Read the model definition and answer for the solid it produces. Units are mm, in the model's axes. A direction names the side the tool comes from. Coordinates: 2 decimals unless noted, no trailing zeros. Loops run counter-clockwise (first coordinate to the right, second up) from the corner with the lowest first, then second, coordinate; pieces in that order, holes last. Notation, with made-up numbers: (-12.75, 55) - (-8.75, 55) arc R29 cw to (-8.75, 88) - close; hole circle Ø11 at (27.25, -36). An arc over 180 degrees is marked (long way). One line per question, with ' | ' between items. Start each with the question number.
```python
from build123d import *

# Parameters (mm, degrees)
F0_R     = 2
F1_DEPTH = 20
F2_W     = 1
F2_H     = 5.5
F3_DEPTH = 10
F4_R     = 1.5
F5_DEPTH = 26.301
F6_SIZE  = 0.5
F7_R     = 1
F9_DEPTH = 3


with BuildPart() as f1:
    # F0 (on Top) → F1 (new body)
    with BuildSketch(Plane.XY):
        with BuildLine():
            Line((0, 3), (0, 0))
            Line((0, 0), (10, 0))
            ThreePointArc((10, 0), (23.15, 13.15), (10, 26.3))
            Line((10, 26.3), (0, 26.3))
            Line((0, 26.3), (0, 23.3))
            Line((0, 23.3), (10, 23.3))
            Line((10, 23.3), (10, 3))
            Line((10, 3), (0, 3))
        make_face()
        with Locations((17, 13.15)):
            Circle(F0_R, mode=Mode.SUBTRACT)
    extrude(amount=F1_DEPTH)

    # F2 (on face) → F3 (join, through all)
    with BuildSketch(Plane(origin=(10, 0, 0), x_dir=(0, -1, 0), z_dir=(-1, 0, 0))):
        with Locations((-22.8, 10)):
            Rectangle(F2_W, F2_H)
        with Locations((-3.5, 10)):
            Rectangle(F2_W, F2_H)
    extrude(amount=F3_DEPTH)

    # F4 (on face) → F5 (cut, through all)
    with BuildSketch(Plane.XZ):
        with Locations((5, 10)):
            Circle(F4_R)
    extrude(amount=-F5_DEPTH, mode=Mode.SUBTRACT)

    # F6
    f6_edges = [f1.edges().sort_by_distance(p)[0] for p in [
        (15, 13.15, 0),
    ]]
    chamfer(f6_edges, length=F6_SIZE)

    # F7
    f7_edges = [f1.edges().sort_by_distance(p)[0] for p in [
        (23.15, 13.15, 20),
        (23.15, 13.15, 0),
        (0, 0, 10),
        (0, 26.3, 10),
    ]]
    fillet(f7_edges, radius=F7_R)

    # F8 (on face) → F9 (cut)
    with BuildSketch(Plane.XY.offset(20)):
        Polygon((20.75, 10.984936), (20.75, 15.315064), (17, 17.480127), (13.25, 15.315064), (13.25, 10.984936), (17, 8.819873), align=None)
    extrude(amount=-F9_DEPTH, mode=Mode.SUBTRACT)


solid = f1.part
```
1) Which of the six approach directions +Z, -Z, +X, -X, +Y, -Y give full straight-line access (tool end or side, diameter ignored) to faces 4 (the flat face through (5.1, 3.5, 12.75)), 5 (the flat face through (5, 23.3, 4)), 6 (the flat face through (0, 24, 10)), 7 (the flat face through (13.25, 13, 19)), 8 (the flat face through (6.2, 4, 11.2))?
2) The mould has two halves that part along X. Classify faces 1 (the flat face through (0, 2, 10)), 2 (the flat face through (15.15, 16.41, 18.52)), 3 (the flat face through (5, 3, 16)): released by +X, released by -X, zero draft, split by the parting line, or undercut.
3) Given pin 1 Ø1 at (y, z) = (7.5, 14.5) entering from +X; pin 2 Ø5 at (x, z) = (5, 10) entering from -Y; pin 3 Ø2.5 at (x, z) = (5, 10) entering from -Y; pin 4 Ø4.5 at (x, y) = (17, 13.15) entering from -Z, each flat-ended and moving along its own axis, determine where each tip first touches the part or whether it passes through.
4) Find the intervals of material crossed by line 1 along Z through (x, y) = (5, 1.6); line 2 along X through (y, z) = (13.15, 13); line 3 along Y through (x, z) = (5.75, 2), in increasing order. Write a range as from..to.
5) The part is cut by section C-C on z = 2.25. Write down the section's boundary in (x, y), and give its area (3 significant figures).
6) The part is cut by section D-D on x = 5. Write down the section's boundary in (y, z).
7) The part is cut by section A-A on x = 2. Write down the section's boundary in (y, z).
8) The part is cut by section B-B on y = 13.15. Write down the section's boundary in (x, z), and give its area (3 significant figures).
Answer below:
1) face 4: +Z, -X | face 5: -Z, -X | face 6: +Z, -Z, -X, +Y, -Y | face 7: +Z | face 8: +Z, -Z, -X
2) face 1: released by -X | face 2: undercut | face 3: zero draft
3) pin 1: x = 22.1 | pin 2: y = 0 | pin 3: through | pin 4: z = 0.25
4) line 1: 0..8.5, 11.5..20 | line 2: 10..15, 19..23.15 | line 3: 0..3, 23.3..26.3
5) outline: (0, 1) arc R1 ccw to (1, 0) - (10, 0) arc R13.15 ccw to (10, 26.3) - (1, 26.3) arc R1 ccw to (0, 25.3) - (0, 23.3) - (10, 23.3) - (10, 3) - (0, 3) - close; hole circle Ø4 at (17, 13.15) | area: 319 mm2
6) outline: (0, 1) arc R1 ccw to (1, 0) - (3, 0) - (3, 7.25) - (4, 7.25) - (4, 8.5) - (0, 8.5) - close; (0, 11.5) - (4, 11.5) - (4, 12.75) - (3, 12.75) - (3, 20) - (1, 20) arc R1 ccw to (0, 19) - close; (22.3, 7.25) - (23.3, 7.25) - (23.3, 0) - (25.3, 0) arc R1 ccw to (26.3, 1) - (26.3, 8.5) - (22.3, 8.5) - close; (22.3, 11.5) - (26.3, 11.5) - (26.3, 19) arc R1 ccw to (25.3, 20) - (23.3, 20) - (23.3, 12.75) - (22.3, 12.75) - close
7) outline: (0, 1) arc R1 ccw to (1, 0) - (3, 0) - (3, 7.25) - (4, 7.25) - (4, 12.75) - (3, 12.75) - (3, 20) - (1, 20) arc R1 ccw to (0, 19) - close; (22.3, 7.25) - (23.3, 7.25) - (23.3, 0) - (25.3, 0) arc R1 ccw to (26.3, 1) - (26.3, 19) arc R1 ccw to (25.3, 20) - (23.3, 20) - (23.3, 12.75) - (22.3, 12.75) - close
8) outline: (10, 0) - (14.5, 0) - (15, 0.5) - (15, 17) - (13.25, 17) - (13.25, 20) - (10, 20) - close; (19, 0.5) - (19.5, 0) - (22.15, 0) arc R1 ccw to (23.15, 1) - (23.15, 19) arc R1 ccw to (22.15, 20) - (20.75, 20) - (20.75, 17) - (19, 17) - close | area: 172 mm2
